Work out the finished part from the listing and answer in its coordinate system (mm). A direction names the side the tool comes from. Round coordinates to 2 decimals unless told otherwise and drop trailing zeros. Loops run counter-clockwise (first coordinate to the right, second up) from the corner with the lowest first, then second, coordinate; pieces in that order, holes last. Notation, with made-up numbers: (27, 28.25) - (80, 28.25) arc R10 cw to (80, 41.25) - close; hole circle Ø1 at (-11.5, 46.25). An arc over 180 degrees is marked (long way). Return JSON: item names as keys, results as strings.
from build123d import *

# Parameters (mm, degrees)
F0_W     = 8.6
F0_H     = 4.1
F0_W_2   = 9.2
F0_H_2   = 11.5
F1_DEPTH = 1.5
F2_D     = 5.2
F2_DEPTH = 2
F2_TIP   = 1.5622376095
F3_D     = 7
F3_DEPTH = 2
F3_TIP   = 2.1030121666
F4_D     = 5.3
F4_DEPTH = 2
F4_TIP   = 1.5922806404


# Not quite as in the source:
# - a feature names something its author has since deleted; it is built from what else it names


with BuildPart() as f1:
    # F0 (on Top) → F1 (new body)
    with BuildSketch(Plane.XY):
        with BuildLine():
            Line((-37.75, -21), (37.75, -21))
            ThreePointArc((37.75, -21), (42.6997474683, -18.9497474683), (44.75, -14))
            Line((44.75, -14), (44.75, 14))
            ThreePointArc((44.75, 14), (42.6997474683, 18.9497474683), (37.75, 21))
            Line((37.75, 21), (-37.75, 21))
            ThreePointArc((-37.75, 21), (-42.6997474683, 18.9497474683), (-44.75, 14))
            Line((-44.75, 14), (-44.75, -14))
            ThreePointArc((-44.75, -14), (-42.6997474683, -18.9497474683), (-37.75, -21))
        make_face()
        with Locations((-5.25, -14.65)):
            Rectangle(F0_W, F0_H, mode=Mode.SUBTRACT)
        with Locations((-19.43, -5.25)):
            Rectangle(F0_W_2, F0_H_2, mode=Mode.SUBTRACT)
    extrude(amount=F1_DEPTH)

    # F2
    with Locations(Plane(origin=(0, 0, 0), x_dir=(1, 0, 0), z_dir=(0, 0, -1))):
        with Locations((18.75, 7), (-28.75, 7)):
            Hole(F2_D / 2, depth=F2_DEPTH)
            with Locations((0, 0, -(F2_DEPTH + F2_TIP / 2))):  # 118° drill point
                Cone(0, F2_D / 2, F2_TIP, mode=Mode.SUBTRACT)

    # F3
    with Locations(Plane(origin=(0, 0, 0), x_dir=(1, 0, 0), z_dir=(0, 0, -1))):
        with Locations((7.55, 7)):
            Hole(F3_D / 2, depth=F3_DEPTH)
            with Locations((0, 0, -(F3_DEPTH + F3_TIP / 2))):  # 118° drill point
                Cone(0, F3_D / 2, F3_TIP, mode=Mode.SUBTRACT)

    # F4
    with Locations(Plane(origin=(0, 0, 0), x_dir=(1, 0, 0), z_dir=(0, 0, -1))):
        with Locations((-30.2482247353, -5.4), (-21.9932247353, -5.4), (-13.7382247353, -5.4), (-5.4832247353, -5.4), (2.7717752647, -5.4), (11.0267752647, -5.4), (19.2817752647, -5.4)):
            Hole(F4_D / 2, depth=F4_DEPTH)
            with Locations((0, 0, -(F4_DEPTH + F4_TIP / 2))):  # 118° drill point
                Cone(0, F4_D / 2, F4_TIP, mode=Mode.SUBTRACT)


solid = f1.part
1) Section A-A (y = -1) is taken. Give the vertices of the cut face in (x, z).
Verdict:
{"outline": "(-44.75, 0) - (-24.03, 0) - (-24.03, 1.5) - (-44.75, 1.5) - close; (-14.83, 0) - (44.75, 0) - (44.75, 1.5) - (-14.83, 1.5) - close"}
2) Section D-D (z = 0.4) is taken. Count the separate pieces of the cut face and the enclosed holes in it, and give its area (3 significant figures).
Verdict:
{"separate pieces": "1", "enclosed holes": "12", "area": "3,340 mm2"}
3) Find the intervals of material crossed by L1, parallel to Y at x = -1.5, z = 1; L2, parallel to Y at x = 5, z = 0.35; L3, parallel to Y at x = 7.55, z = 0.5, in increasing order.
Verdict:
{"L1": "y = -21 to -16.7, -12.6 to 21", "L2": "y = -21 to -9.4, -4.6 to 3.97, 6.83 to 21", "L3": "y = -21 to -10.5, -3.5 to 21"}
4) A tool of negligible diameter and unlimited length cuts with its end or side. For faces 5 (the cylindrical face through (42.75, 18.9, 0.74)), 6 (the flat face through (-5, -16.7, 1)), from which of +Z, -Z, +X, -X, +Y, -Y can it reach the whole face along a straight path? Write none if from no direction.
Verdict:
{"face 5": "+Z, -Z, +X, +Y", "face 6": "+Z, -Z"}
5) Section C-C (y = -7) is taken. Give the vertices of the cut face in (x, z), and give its area (4 significant figures).
Verdict:
{"outline": "(-44.75, 0) - (-31.35, 0) - (-31.35, 1.5) - (-44.75, 1.5) - close; (-26.15, 0) - (-24.03, 0) - (-24.03, 1.5) - (-26.15, 1.5) - close; (-14.83, 0) - (4.05, 0) - (4.05, 1.5) - (-14.83, 1.5) - close; (11.05, 0) - (16.15, 0) - (16.15, 1.5) - (11.05, 1.5) - close; (21.35, 0) - (44.75, 0) - (44.75, 1.5) - (21.35, 1.5) - close", "area": "94.35 mm2"}
6) Determine the mould class of faces 1 (the cylindrical face through (42.65, -19, 0.74)), 2 (the flat face through (-1, 0, 1.5)), 3 (the flat face through (-24.03, -5, 1)), 4 (the flat face through (-19, -11, 1)) for opening direction Y: pulls with the +Y half, pulls with the -Y half, needs draft (parallel to the pull), parting line crosses it, or undercut.
Verdict:
{"face 1": "pulls with the -Y half", "face 2": "needs draft", "face 3": "undercut", "face 4": "undercut"}
7) Section B-B (x = 7.55) is taken. Give the vertices of the cut face in (y, z).
Verdict:
{"outline": "(-21, 0) - (-10.5, 0) - (-10.5, 1.5) - (-21, 1.5) - close; (-3.5, 0) - (21, 0) - (21, 1.5) - (-3.5, 1.5) - close"}
8) A flat-ended cylindrical pin translates along its axis: pin 1 (4 mm diameter, centred on x = -5.48, y = 5.4, fed in from +Z). Find the tip coordinate at first contact, or state that the pin passes through.
Verdict:
{"pin 1": "passes through"}
